Autodesk Inventor part; units mm, degrees
ref_plane "YZ Plane" through (0, 0, 0) normal (1, 0, 0) x (0, 1, 0)
ref_plane "XZ Plane" through (0, 0, 0) normal (0, 1, 0) x (-1, 0, 0)
ref_plane "XY Plane" through (0, 0, 0) normal (0, 0, 1) x (1, 0, 0)
sketch "Sketch1" plane through (0, 0, 0) normal (0, 1, 0) x (-1, 0, 0)
  circle A0 centre (0, 0) radius 3.175
  dimension "d0" = 6.35
extrude "Extrusion1" add sketch "Sketch1" along normal blind 101.6
sketch "Sketch2" plane through (0, 101.6, 0) normal (0, 1, 0) x (1, 0, 0)
  line L0 (6.35, -12.7) -> (-6.35, -12.7)
  line L1 (-6.35, -12.7) -> (-6.35, 12.7)
  line L2 (-6.35, 12.7) -> (6.35, 12.7)
  line L3 (6.35, 12.7) -> (6.35, -12.7)
  line L4 (6.35, -12.7) -> (-6.35, 12.7) construction
  line L5 (-6.35, -12.7) -> (6.35, 12.7) construction
  point P0 (0, 0)
  dimension "d3" = 12.7
  dimension "d4" = 25.4
extrude "Extrusion2" add sketch "Sketch2" along normal blind 3.175
sketch "Sketch3" plane through (0, 104.775, 0) normal (0, 1, 0) x (1, 0, 0)
  point P0 (0, 0)
sketch "Sketch4" plane through (0, 104.775, 0) normal (0, 1, 0) x (1, 0, 0)
  line L0 (6.35, -12.7) -> (6.35, 12.7)
  line L1 (-6.35, -12.7) -> (6.35, -12.7)
  line L2 (6.35, -12.7) -> (6.35, -9.525)
  line L3 (6.35, -9.525) -> (-6.35, -9.525)
  line L4 (-6.35, -9.525) -> (-6.35, -12.7)
  line L5 (-6.35, 12.7) -> (6.35, 12.7)
  line L6 (6.35, 12.7) -> (6.35, 9.525)
  line L7 (6.35, 9.525) -> (-6.35, 9.525)
  line L8 (-6.35, 9.525) -> (-6.35, 12.7)
  line L9 (6.35, 12.7) -> (-6.35, 12.7)
  point P0 (0, 0)
  dimension "d7" = 3.175
  dimension "d8" = 3.175
  dimension "d9" = 0
extrude "Extrusion3" add sketch "Sketch4" along normal blind 15.875
sketch "Sketch5" plane through (6.35, 101.6, -12.7) normal (0, 0, -1) x (-1, 0, 0)
  circle A0 centre (6.35, 12.7) radius 3.175
  line L0 (12.7, 0) -> (0, 0)
  point P0 (6.35, -101.6)
  dimension "d12" = 6.35
  dimension "d13" = 12.7
extrude "Extrusion4" cut sketch "Sketch5" against normal blind 50.8
properties part number "PC3.5-ROD"
Input: part model. Units: mm. Frame: model coordinates. A direction names the side the tool comes from. Give positions to 0.01 mm unless a question says otherwise; leave off trailing zeros. Loops run counter-clockwise (first coordinate to the right, second up) from the corner with the lowest first, then second, coordinate; pieces in that order, holes last. Notation, with made-up numbers: (-15, 78.25) -> (2, 78.25) arc R20 ccw to (2, 83.25) -> close; hole circle Ø4 at (-32.75, 16). An arc over 180 degrees is marked (long way). Answer as a JSON object with one key per item and string values. Group by question number.
Item 1: Pull-direction query (X, two-part tool) for faces 4 (the flat face through (0.1, 110.8, 9.525)), 5 (the flat face through (-6.35, 104.6, 0.2)), 6 (the cylindrical face through (0.69, 111.2, -11.13)); classes: released by +X, released by -X, zero draft, split by the parting line, or undercut.
Item 2: Cut plane B-B, the plane z = 0. Return the cut outline in (x, y) (3 decimals), and give its area (3 significant figures).
Item 3: Pin query (flat end, axial travel): P1, Ø1, axis at y = 35, z = 2, coming from the -X side; P2, Ø12, axis at y = 47, z = -1.5, coming from the -X side (3 decimals); P3, Ø4, axis at x = 4, y = 96.5, coming from the -Z side. Return the tip coordinate at first contact, or that it passes through.
Item 4: Reachability of faces 1 (the flat face through (-2, 101.6, -3)), 2 (the flat face through (0.1, 110.8, -9.525)), 3 (the flat face through (0, 120.65, -11)) from +Z, -Z, +X, -X, +Y, -Y: full face, straight path, thin tool, end or side. Return the list, or none.
Item 5: Cut plane D-D, the plane y = 35. Return the cut outline in (x, z) (3 decimals).
Item 6: Line query: probe 1 along Y at (x, z) = (0, 11.8) (3 decimals); probe 2 along Z at (x, y) = (-4.25, 112.5) (3 decimals); probe 3 along Y at (x, z) = (3.5, 3.75) (3 decimals). Output: solid intervals per line, ascending.
Item 7: Cut plane C-C, the plane x = 0. Return the cut outline in (y, z) (3 decimals), and give its area (3 significant figures).
Item 8: Cut plane A-A, the plane y = 114.3. Return the cut outline in (x, z) (3 decimals).
Checks:
{
 "1": {"face 4": "zero draft", "face 5": "released by -X", "face 6": "undercut"},
 "2": {"outline": "(-6.35, 101.6) -> (-3.175, 101.6) -> (-3.175, 0) -> (3.175, 0) -> (3.175, 101.6) -> (6.35, 101.6) -> (6.35, 104.775) -> (-6.35, 104.775) -> close", "area": "685 mm²"},
 "3": {"P1": "stops at x = -2.8", "P2": "stops at x = -3.175", "P3": "stops at z = -2.47"},
 "4": {"face 1": "-Y", "face 2": "+X, -X, +Y", "face 3": "+Z, -Z, +X, -X, +Y"},
 "5": {"outline": "circle Ø6.35 at (0, 0)"},
 "6": {"probe 1": "y = 101.6 to 111.125, 117.475 to 120.65", "probe 2": "z = -12.7 to -9.525, 9.525 to 12.7", "probe 3": "y = 101.6 to 104.775"},
 "7": {"outline": "(0, -3.175) -> (101.6, -3.175) -> (101.6, -12.7) -> (111.125, -12.7) -> (111.125, -9.525) -> (104.775, -9.525) -> (104.775, 9.525) -> (111.125, 9.525) -> (111.125, 12.7) -> (101.6, 12.7) -> (101.6, 3.175) -> (0, 3.175) -> close; (117.475, -12.7) -> (120.65, -12.7) -> (120.65, -9.525) -> (117.475, -9.525) -> close; (117.475, 9.525) -> (120.65, 9.525) -> (120.65, 12.7) -> (117.475, 12.7) -> close", "area": "786 mm²"},
 "8": {"outline": "(-6.35, -12.7) -> (-3.175, -12.7) -> (-3.175, -9.525) -> (-6.35, -9.525) -> close; (-6.35, 9.525) -> (-3.175, 9.525) -> (-3.175, 12.7) -> (-6.35, 12.7) -> close; (3.175, -12.7) -> (6.35, -12.7) -> (6.35, -9.525) -> (3.175, -9.525) -> close; (3.175, 9.525) -> (6.35, 9.525) -> (6.35, 12.7) -> (3.175, 12.7) -> close"}
}
